The model under review builds one solid part; all positions refer to its coordinate system, in mm. A direction names the side the tool comes from. Give positions to 0.01 mm unless a question says otherwise; leave off trailing zeros. Loops run counter-clockwise (first coordinate to the right, second up) from the corner with the lowest first, then second, coordinate; pieces in that order, holes last. Notation, with made-up numbers: M 84,62.25 L 133,62.25 A10 ccw 133,67.25 Z; hole C -10,-14 d6. An arc over 180 degrees is marked long. Write item = value, one per line. Start each with the question number.
1. Wall thickness on line 1 along X through (y, z) = (2.65, 27); line 2 along X through (y, z) = (0.6, 12); line 3 along Z through (x, y) = (0.5, 3.65): over which ranges is each line inside the solid? List them lowest first. Write a range as from..to.
2. Draft analysis for pull direction Z (two halves, no side actions). For faces 1 (the face through (-15.376, 2.465, -15.737)), 2 (the face through (35.4, 2.54, 35.43)), 3 (the face through (36, 2, 0)), state which applies: pulls with the +Z half, pulls with the -Z half, needs draft (parallel to the pull), parting line crosses it, or undercut.
3. We need section D-D on z = -27. Give the boundary of the cut face in (x, y), then the cut area to 3 significant figures.
4. We need section A-A on y = 2.8. Give the boundary of the cut face in (x, z), then the cut area to 3 significant figures.
5. We need section B-B on x = 5.5. Give the boundary of the cut face in (y, z), then the cut area to 3 significant figures.
6. For faces 4 (the face through (35.4, 2.54, -35.43)), 5 (the face through (13.81, 2.46, -20.88)), list the 3-axis set-ups (+Z, -Z, +X, -X, +Y, -Y) from which the entire face can be reached by the end or side of a thin tool; tool diameter is ignored.
7. We need section C-C on z = -7. Give the boundary of the cut face in (x, y), then the cut area to 3 significant figures.
from build123d import *

# Parameters (mm, degrees)
SKETCH1_W           = 72
SKETCH1_H           = 72
SKETCH1_R           = 2.95
BOSS_EXTRUDE1_DEPTH = 5
FILLET1_R           = 2


with BuildPart() as part:
    # Sketch1 → Boss-Extrude1 (new body)
    with BuildSketch(Plane(origin=(0, 0, 0), x_dir=(1, 0, 0), z_dir=(0, 1, 0))):
        Rectangle(SKETCH1_W, SKETCH1_H)
        with Locations(Location((-27, 27, 0), (0, 0, 270))):
            Circle(SKETCH1_R, mode=Mode.SUBTRACT)
        with Locations(Location((27, -27, 0), (0, 0, 270))):
            Circle(SKETCH1_R, mode=Mode.SUBTRACT)
        with Locations(Location((-27, -27, 0), (0, 0, 270))):
            Circle(SKETCH1_R, mode=Mode.SUBTRACT)
        with Locations(Location((27, 27, 0), (0, 0, 270))):
            Circle(SKETCH1_R, mode=Mode.SUBTRACT)
        Polygon((-28.461047943, -2.651650429), (-2.651650429, -28.461047943), (2.651650429, -28.461047943), (28.461047943, -2.651650429), (28.461047943, 2.651650429), (19.091883092, 12.02081528), (22.627416998, 15.556349186), (15.556349186, 22.627416998), (12.02081528, 19.091883092), (2.651650429, 28.461047943), (-2.651650429, 28.461047943), (-28.461047943, 2.651650429), align=None, mode=Mode.SUBTRACT)
    extrude(amount=BOSS_EXTRUDE1_DEPTH)

    # Fillet1
    fillet1_edges = [part.edges().sort_by_distance(p)[0] for p in [
        (36, 2.5, 36),
        (-36, 2.5, 36),
        (-36, 2.5, -36),
        (36, 2.5, -36),
    ]]
    fillet(fillet1_edges, radius=FILLET1_R)


solid = part.part
Final values:
q1.line_1 = -36..-29.95, -24.05..-4.11, 4.11..24.05, 29.95..36
q1.line_2 = -36..-19.11, 19.11..36
q1.line_3 = -36..-28.46, 28.46..36
q2.face_1 = undercut
q2.face_2 = pulls with the +Z half
q2.face_3 = needs draft
q3.outline = M -36,0 L -29.95,0 L -29.95,5 L -36,5 Z; M -24.05,0 L -4.11,0 L -4.11,5 L -24.05,5 Z; M 4.11,0 L 24.05,0 L 24.05,5 L 4.11,5 Z; M 29.95,0 L 36,0 L 36,5 L 29.95,5 Z
q3.area = 260 mm²
q4.outline = M -36,-34 A2 ccw -34,-36 L 34,-36 A2 ccw 36,-34 L 36,34 A2 ccw 34,36 L -34,36 A2 ccw -36,34 Z; hole C -27,-27 d5.9; hole C -27,27 d5.9; hole M -28.46,-2.65 L -2.65,-28.46 L 2.65,-28.46 L 12.02,-19.09 L 15.56,-22.63 L 22.63,-15.56 L 19.09,-12.02 L 28.46,-2.65 L 28.46,2.65 L 2.65,28.46 L -2.65,28.46 L -28.46,2.65 Z; hole C 27,-27 d5.9; hole C 27,27 d5.9
q4.area = 3,110 mm²
q5.outline = M 0,-36 L 5,-36 L 5,-25.61 L 0,-25.61 Z; M 0,25.61 L 5,25.61 L 5,36 L 0,36 Z
q5.area = 104 mm²
q6.face_4 = -Z, +X, +Y, -Y
q6.face_5 = +Y, -Y
q7.outline = M -36,0 L -24.11,0 L -24.11,5 L -36,5 Z; M 24.11,0 L 36,0 L 36,5 L 24.11,5 Z
q7.area = 119 mm²
